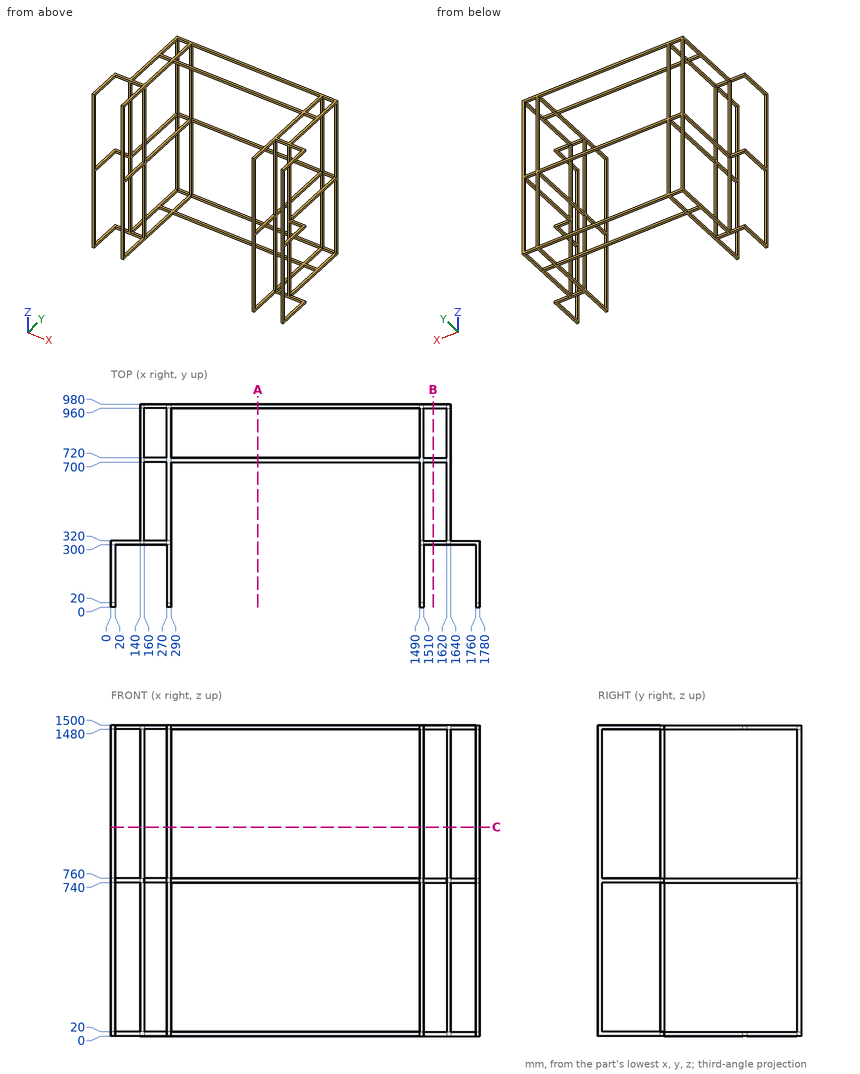
Design review of the part shown in the three views and the two pictorial views. Dimensions are in mm from the part's minimum x, y and z. Give positions to 0.01 mm unless a question says otherwise; leave off trailing zeros. Loops run counter-clockwise (first coordinate to the right, second up) from the corner with the lowest first, then second, coordinate; pieces in that order, holes last. Notation, with made-up numbers: M 3,50.25 L 14,50.25 A10 ccw 14,56.25 Z; hole C 73.25,84 d5. An arc over 180 degrees is marked long. Answer as a JSON object with one key per item and string values.
Item 1: Wall thickness on line 1 along Z through (x, y) = (1509, 282.5); line 2 along X through (y, z) = (319, 673): over which ranges is each line inside the solid? List them lowest first.
Output values:
{"line 1": "z = 0 to 20, 740 to 760, 1480 to 1500", "line 2": "x = 140 to 160, 270 to 290, 1490 to 1510, 1620 to 1640"}
Item 2: We need section C-C (z = 1008). Count the separate pieces of the cut face and the enclosed holes in it, and give its area (3 significant figures).
Output values:
{"separate pieces": "12", "enclosed holes": "0", "area": "4,800 mm2"}
Item 3: We need section B-B (x = 1554). State the section outline as (y, z) points, and give its area (3 significant figures).
Output values:
{"outline": "M 300,0 L 320,0 L 320,20 L 300,20 Z; M 300,1480 L 320,1480 L 320,1500 L 300,1500 Z; M 700,0 L 720,0 L 720,20 L 700,20 Z; M 700,1480 L 720,1480 L 720,1500 L 700,1500 Z; M 960,0 L 980,0 L 980,20 L 960,20 Z; M 960,740 L 980,740 L 980,760 L 960,760 Z; M 960,1480 L 980,1480 L 980,1500 L 960,1500 Z", "area": "2,800 mm2"}
Item 4: We need section A-A (x = 709). State the section outline as (y, z) points.
Output values:
{"outline": "M 700,0 L 720,0 L 720,20 L 700,20 Z; M 700,1480 L 720,1480 L 720,1500 L 700,1500 Z; M 960,0 L 980,0 L 980,20 L 960,20 Z; M 960,740 L 980,740 L 980,760 L 960,760 Z; M 960,1480 L 980,1480 L 980,1500 L 960,1500 Z"}
Item 5: For P1, Ø6, axis at x = 217, z = 15, coming from the -Y side; P2, Ø10, axis at x = 749, z = 12, coming from the -Y side; P3, Ø6, axis at x = 39.5, z = 10.5, coming from the +Y side, all flat-tipped, find the tip position at first contact; note any pin that passes through.
Output values:
{"P1": "stops at y = 300", "P2": "stops at y = 700", "P3": "stops at y = 320"}
